```python
from build123d import *

# Parameters (mm, degrees)
ESQUISSE1_R             = 30
BOSS_EXTRU_1_DEPTH      = 35
ESQUISSE2_R             = 2
ENL_V_MAT_EXTRU_1_DEPTH = 10
BOSS_EXTRU_2_START      = -2
ESQUISSE3_R             = 33
ESQUISSE3_R_2           = 30
BOSS_EXTRU_2_DEPTH      = 30


with BuildPart() as part:
    # Esquisse1 → Boss.-Extru.1 (new body)
    with BuildSketch(Plane.XY):
        Circle(ESQUISSE1_R)
    extrude(amount=BOSS_EXTRU_1_DEPTH)

    # Esquisse2 → Enlèv. mat.-Extru.1 (cut)
    with BuildSketch(Plane(origin=(0, 0, 0), x_dir=(-1, 0, 0), z_dir=(0, 0, -1))):
        with Locations((0, 8)):
            Circle(ESQUISSE2_R)
        with Locations((8, 0)):
            Circle(ESQUISSE2_R)
        with Locations((0, -8)):
            Circle(ESQUISSE2_R)
        with Locations((-8, 0)):
            Circle(ESQUISSE2_R)
        Circle(ESQUISSE2_R)
    extrude(amount=-ENL_V_MAT_EXTRU_1_DEPTH, mode=Mode.SUBTRACT)

    # Esquisse3 → Boss.-Extru.2 (add)
    with BuildSketch(Plane(origin=(0, 0, 0), x_dir=(-1, 0, 0), z_dir=(0, 0, -1)).offset(BOSS_EXTRU_2_START)):
        Circle(ESQUISSE3_R)
        Circle(ESQUISSE3_R_2, mode=Mode.SUBTRACT)
    extrude(amount=-BOSS_EXTRU_2_DEPTH)


solid = part.part
```
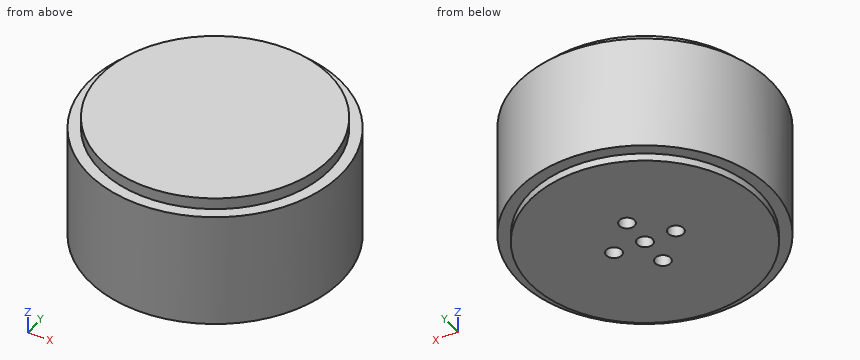
For this review, take the finished solid that the model builds, in its own axes (mm). Round coordinates to 2 decimals unless told otherwise and drop trailing zeros. Write each loop counter-clockwise with the first axis right and the second up, starting at its lowest first coordinate (ties: lowest second). Pieces come first, ordered by that corner, then holes.
1) Take a section at B-B on z = 7. Give the boundary of the cut face in (x, y).
Answer below:
outline: circle Ø66 at (0, 0); hole circle Ø4 at (-8, 0); hole circle Ø4 at (0, -8); hole circle Ø4 at (0, 0); hole circle Ø4 at (0, 8); hole circle Ø4 at (8, 0)
2) Take a section at A-A on y = 0. Give the boundary of the cut face in (x, z).
Answer below:
outline: (-33, 2) - (-30, 2) - (-30, 0) - (-10, 0) - (-10, 10) - (-6, 10) - (-6, 0) - (-2, 0) - (-2, 10) - (2, 10) - (2, 0) - (6, 0) - (6, 10) - (10, 10) - (10, 0) - (30, 0) - (30, 2) - (33, 2) - (33, 32) - (30, 32) - (30, 35) - (-30, 35) - (-30, 32) - (-33, 32) - close
3) For line 1 along Y through (x, z) = (0, 6.5); line 2 along Y through (x, z) = (8, 4); line 3 along X through (y, z) = (27, 24.5), list the stretches that pass through material, from the lowest coordinate up.
Answer below:
line 1: y = -33 to -10, -6 to -2, 2 to 6, 10 to 33
line 2: y = -32.02 to -2, 2 to 32.02
line 3: x = -18.97 to 18.97
4) Take a section at D-D on z = 17.5. Give the boundary of the cut face in (x, y).
Answer below:
outline: circle Ø66 at (0, 0)
5) Insertion check: pin 1 Ø3 at (x, y) = (-8.5, -1) entering from -Z; pin 2 Ø1.2 at (x, y) = (7.5, 0) entering from -Z; pin 3 Ø12 at (x, z) = (-14, 24.5) entering from +Y; pin 4 Ø2 at (y, z) = (3, 7) entering from +X. Each pin has a flat end and moves straight along its axis. Give the tip position at first contact, or say it passes through.
Answer below:
pin 1: stops at z = 0
pin 2: stops at z = 10
pin 3: stops at y = 32.02
pin 4: stops at x = 32.94
